Read the model definition and answer for the solid it produces. Units are mm, in the model's axes. Face numbers are marked on the shaded views. A direction names the side the tool comes from. Coordinates: 2 decimals unless noted, no trailing zeros. Order: outer loops, then holes, each group sorted by start corner. A loop starts at its lowest first (then second) coordinate and runs counter-clockwise, first axis right, second up. Notation, with made-up numbers: M 25.25,64.25 L 44.25,64.25 A21 ccw 44.25,72.25 Z; hole C -17.5,-34.75 d6. An arc over 180 degrees is marked long. Put each result on its own line as item: value.
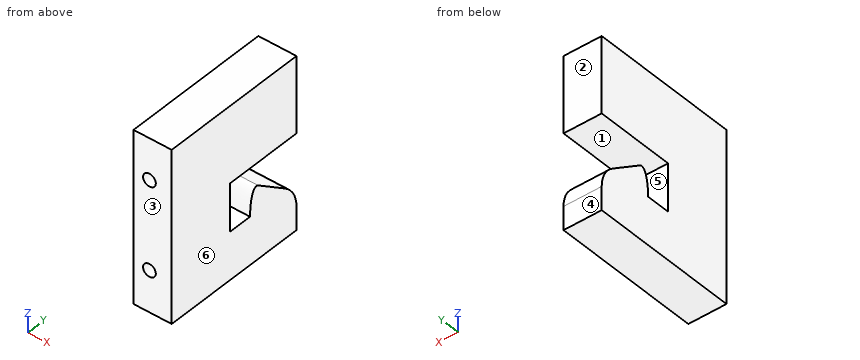
Solid Edge part; units mm, degrees
sketch "Sketch1" plane through (0, 0, 0) normal (1, 0, 0) x (0, 1, 0)
  line L0 (-23.5, -27) -> (23.5, -27)
  line L1 (23.5, -27) -> (23.5, 27)
  line L2 (23.5, 27) -> (-23.5, 27)
  line L3 (-23.5, 27) -> (-23.5, -27)
  dimension "D1" = 23.5
  dimension "D2" = 23.5
extrude "Protrusion1" add sketch "Sketch1" along normal mid plane 12
hole "Bohrung_1" at (-1, -23.5, 14) direction (0, 1, 0) diameter 4 depth 6
hole "Hole1" at (-1, -23.5, -14) direction (0, 1, 0) diameter 4 depth 6
sketch "Sketch2" plane through (6, 0, 0) normal (1, 0, 0) x (0, 1, 0)
  line L0 (23.5, -14.5) -> (6, -2)
  line L1 (6, -2) -> (6, -12)
  line L2 (6, -12) -> (-1.5, -12)
  line L3 (-1.5, -12) -> (-1.5, 3)
  line L4 (-1.5, 3) -> (23.5, 3)
  line L5 (23.5, 3) -> (23.5, -14.5)
  dimension "D1" = 1.5
  dimension "D2" = 6
  dimension "D3" = 1.5
  dimension "D4" = 6
extrude "Extrusionsausschnitt_1" cut sketch "Sketch2" against normal blind 135.5146
sketch "Sketch3" plane through (6, 0, 0) normal (1, 0, 0) x (0, 1, 0)
  spline S0 degree 3 poles (6, -12) (6.0478, -6.0252) (7.4729, -2.7697) (9.3635, -4.4025) knots 0 0 0 0 1 1 1 1
  line L0 (9.3635, -4.4025) -> (9.8723, -3.23)
  line L1 (9.8723, -3.23) -> (5.7538, -1.5265)
  line L2 (5.7538, -1.5265) -> (6, -12)
extrude "Extrusionsausschnitt_3" cut sketch "Sketch3" along normal mid plane 89.7467
fillet "Verrundung_1" radius 10 1 edges at (0, 23.5, -14.5)
Q1. Consider line 1 along Z through (x, y) = (-1, -21.2); line 2 along X through (y, z) = (-19.45, -14); line 3 along Z through (x, y) = (-2, -19.5). Determine where each line is inside the solid, lowest interval first.
Answers below:
line 1: z = -27 to -16, -12 to 12, 16 to 27
line 2: x = -6 to -3, 1 to 6
line 3: z = -27 to -15.73, -12.27 to 12.27, 15.73 to 27
Q2. Find section B-B on z = 14. Write down the section's boundary in (x, y).
Answers below:
outline: M -6,-23.5 L -3,-23.5 L -3,-17.5 L 1,-17.5 L 1,-23.5 L 6,-23.5 L 6,23.5 L -6,23.5 Z
Q3. Given pin 1 (2 mm diameter, centred on x = 4, z = -12.5, fed in from +Y); pin 2 (3 mm diameter, centred on x = -4, z = -6.5, fed in from +Y); pin 3 (2.5 mm diameter, centred on x = -1, z = -14, fed in from -Y), each flat-ended and moving along its own axis, determine where each tip first touches the part or whether it passes through.
Answers below:
pin 1: stops at y = 21.39
pin 2: stops at y = 14.4
pin 3: stops at y = -17.5
Q4. For a pull along Y with two mould halves and no side action, classify the marked faces 3, 4, 5 and 6 as +Y half, -Y half, draft (parallel to the pull), parting line (faces both ways), or undercut.
Answers below:
face 3: -Y half
face 4: +Y half
face 5: undercut
face 6: draft
Q5. Find section A-A on y = 15. Write down the section's boundary in (x, z), plus the area to 3 significant figures.
Answers below:
outline: M -6,-27 L 6,-27 L 6,-8.43 L -6,-8.43 Z; M -6,3 L 6,3 L 6,27 L -6,27 Z
area: 511 mm^2
Q6. Find section C-C on z = -14. Write down the section's boundary in (x, y), plus the area to 3 significant figures.
Answers below:
outline: M -6,-23.5 L -3,-23.5 L -3,-17.5 L 1,-17.5 L 1,-23.5 L 6,-23.5 L 6,21.75 L -6,21.75 Z
area: 519 mm^2
Q7. A tool of negligible diameter and unlimited length cuts with its end or side. For the marked faces 1 and 2, from which of +Z, -Z, +X, -X, +Y, -Y can it reach the whole face along a straight path? Write none if from no direction.
Answers below:
face 1: +X, -X, +Y
face 2: +Z, -Z, +X, -X, +Y
